Input: part model. Units: mm. Frame: model coordinates. A direction names the side the tool comes from. Coordinates: 2 decimals unless noted, no trailing zeros. Loops run counter-clockwise (first coordinate to the right, second up) from the corner with the lowest first, then second, coordinate; pieces in that order, holes last.
Item 1: Section A-A on x = -2.5. Return loops of the section in (y, z), and give its area (3 significant figures).
Item 2: Contact query for flat-ended pins moving along their axis: P1, Ø0.8, axis at y = 2, z = 1, coming from the +X side; P2, Ø1.5, axis at y = -13.25, z = 2.5, coming from the -X side; P3, Ø1.5, axis at x = -41, z = 0.5, coming from the -Y side. Output: stop coordinate, or through.
Item 3: Reachability of faces 1 (the flat face through (60.5, 12, 1)), 2 (the flat face through (62, -7.5, 4)), 3 (the flat face through (-9.92, -5.79, 2.46)) from +Z, -Z, +X, -X, +Y, -Y: full face, straight path, thin tool, end or side. Return the list, or none.
Item 4: Pull-direction query (Z, two-part tool) for faces 4 (the cylindrical face through (11.1, 15.2, 2.5)), 5 (the flat face through (0, -17, 2.5)), 6 (the cylindrical face through (16.22, -14.98, 2.34)); classes: released by +Z, released by -Z, zero draft, split by the parting line, or undercut.
Item 5: Ray query, line 1 along Y through (x, z) = (58.7, 2.5); line 2 along X through (y, z) = (15, 2.7); line 3 along Z through (x, y) = (-15, 14.75). Return the intervals inside material, ascending.
Item 6: Section B-B on x = 11.05. Return loops of the section in (y, z).
Autodesk Inventor part; units mm, degrees
ref_plane "YZ Plane" through (0, 0, 0) normal (1, 0, 0) x (0, 1, 0)
ref_plane "XZ Plane" through (0, 0, 0) normal (0, 1, 0) x (-1, 0, 0)
ref_plane "XY Plane" through (0, 0, 0) normal (0, 0, 1) x (1, 0, 0)
sketch "スケッチ1" plane through (0, 0, 0) normal (0, 0, 1) x (1, 0, 0)
  line L0 (-60.5, 9.6) -> (-60.5, 16.25)
  line L1 (-60.5, 16.25) -> (-20, 16.25)
  line L2 (20, 16.25) -> (60.5, 16.25)
  line L3 (60.5, 16.25) -> (60.5, 9.6)
  line L4 (0, 0) -> (0, 16.25) construction
  line L5 (0, 0) -> (62.5, 0) construction
  line L6 (60.5, 7.5) -> (62.5, 7.5)
  line L7 (62.5, 7.5) -> (62.5, -7.5)
  line L8 (62.5, -7.5) -> (60.5, -7.5)
  line L9 (-20, -16.25) -> (20, -16.25) construction
  line L10 (20, -16.25) -> (20, 16.25) construction
  line L11 (20, 16.25) -> (-20, 16.25) construction
  line L12 (-20, 16.25) -> (-20, -16.25) construction
  line L13 (-20, -16.25) -> (20, 16.25) construction
  line L14 (20, -16.25) -> (-20, 16.25) construction
  line L15 (-60.5, -16.25) -> (60.5, -16.25) construction
  line L16 (60.5, -16.25) -> (60.5, 16.25) construction
  line L17 (60.5, 16.25) -> (-60.5, 16.25) construction
  line L18 (-60.5, 16.25) -> (-60.5, -16.25) construction
  line L19 (-60.5, -16.25) -> (60.5, 16.25) construction
  line L20 (60.5, -16.25) -> (-60.5, 16.25) construction
  arc A0 (60.5, 9.6) -> (60.5, 7.5) centre (60.5, 8.55) ccw
  arc A1 (60.5, -7.5) -> (60.5, -9.6) centre (60.5, -8.55) ccw
  line L21 (60.5, -9.6) -> (60.5, -16.25)
  line L22 (60.5, -16.25) -> (20, -16.25)
  line L23 (20, -16.25) -> (12.1, -16.25)
  line L24 (-20, 16.25) -> (-12.1, 16.25)
  line L25 (-10, 16.25) -> (-10, 18.25)
  line L26 (-10, 18.25) -> (10, 18.25)
  line L27 (10, 18.25) -> (10, 16.25)
  line L28 (20, 16.25) -> (12.1, 16.25)
  arc A2 (-12.1, 16.25) -> (-10, 16.25) centre (-11.05, 16.25) ccw
  arc A3 (10, 16.25) -> (12.1, 16.25) centre (11.05, 16.25) ccw
  line L29 (-60.5, 7.5) -> (-62.5, 7.5)
  line L30 (-62.5, 7.5) -> (-62.5, -7.5)
  line L31 (-62.5, -7.5) -> (-60.5, -7.5)
  arc A4 (-60.5, 7.5) -> (-60.5, 9.6) centre (-60.5, 8.55) ccw
  arc A5 (-60.5, -9.6) -> (-60.5, -7.5) centre (-60.5, -8.55) ccw
  line L32 (-60.5, -9.6) -> (-60.5, -16.25)
  line L33 (-60.5, -16.25) -> (-20, -16.25)
  line L34 (-20, -16.25) -> (-12.1, -16.25)
  line L35 (-10, -16.25) -> (-10, -18.25)
  line L36 (-10, -18.25) -> (10, -18.25)
  line L37 (10, -18.25) -> (10, -16.25)
  arc A6 (-10, -16.25) -> (-12.1, -16.25) centre (-11.05, -16.25) ccw
  arc A7 (12.1, -16.25) -> (10, -16.25) centre (11.05, -16.25) ccw
  line L38 (-16.55, 19.1799) -> (-13.45, 19.1799) construction
  line L39 (-13.45, 19.1799) -> (-13.45, 12.4242) construction
  line L40 (-13.45, 12.4242) -> (-16.55, 12.4242) construction
  line L41 (-16.55, 12.4242) -> (-16.55, 19.1799) construction
  line L42 (-15, 19.1799) -> (-15, 12.4242) construction
  point P0 (0, 18.25)
  point P1 (0, 0)
  dimension "d0" = 1.05
  dimension "d1" = 32.5
  dimension "d2" = 121
  dimension "d3" = 40
  dimension "d23" = 2
  dimension "d30" = 2
  dimension "d34" = 8.75
  dimension "d53" = 20
  dimension "d54" = 3.1
  dimension "d55" = 5
  dimension "d85" = 32.5
extrude "押し出し1" add sketch "スケッチ1" along normal blind 5
sketch "スケッチ2" plane through (0, 0, 0) normal (0, 0, -1) x (-1, 0, 0)
  line L0 (60.5, 9.6) -> (60.5, 16.25)
  line L1 (-60.5, 16.25) -> (-60.5, 9.6)
  line L2 (-68.6427, 17.3125) -> (-60.5, 17.3125)
  line L3 (-60.5, 17.3125) -> (-60.5, -16.751)
  line L4 (-60.5, -16.751) -> (-68.6427, -16.751)
  line L5 (-68.6427, -16.751) -> (-68.6427, 17.3125)
  line L6 (60.5, 21.1805) -> (66.358, 21.1805)
  line L7 (66.358, 21.1805) -> (66.358, -13.6193)
  line L8 (66.358, -13.6193) -> (60.5, -13.6193)
  line L9 (60.5, -13.6193) -> (60.5, 21.1805)
  line L10 (-20, -16.25) -> (-12.1, -16.25)
  line L11 (-17.1371, 25.1848) -> (11.8342, 25.1848)
  line L12 (11.8342, 25.1848) -> (11.8342, 16.25)
  line L13 (11.8342, 16.25) -> (-17.1371, 16.25)
  line L14 (-17.1371, 16.25) -> (-17.1371, 25.1848)
  line L15 (-13.151, -21.5857) -> (17.7795, -21.5857)
  line L16 (17.7795, -21.5857) -> (17.7795, -16.25)
  line L17 (17.7795, -16.25) -> (-13.151, -16.25)
  line L18 (-13.151, -16.25) -> (-13.151, -21.5857)
  line L19 (-12.1, 16.25) -> (-60.5, 16.25)
  line L20 (-60.5, -16.25) -> (-12.1, -16.25)
  point P0 (0, 0)
extrude "押し出し2" cut sketch "スケッチ2" against normal blind 2.5
sketch "スケッチ3" plane through (12.1, 16.25, 0) normal (0, 1, 0) x (1, 0, 0)
  line L0 (-2.1, 0) -> (-2.1, -5)
  line L1 (-2.1, -5) -> (-22.1, -5) construction
  line L2 (-12.1, -5) -> (-12.1, 7.4607) construction
  line L3 (48.4, 0) -> (48.4, -5)
  point P0 (-12.1, 0)
  point P1 (2.9, -2.5)
  point P2 (-27.1, -2.5)
  point P3 (48.4, -2.5)
  dimension "d60" = 5
hole "穴1" at (15, 16.25, 2.5) at (-15, 16.25, 2.5) direction (0, -1, 0) diameter 2.459 depth 2.5
mirror "ミラー1" about plane through (0, 0, 0) normal (0, 1, 0) of "穴1"
sketch "スケッチ4" plane through (60.5, -16.25, 5) normal (1, 0, 0) x (0, 0, -1)
  line L0 (5, 16.25) -> (0, 16.25) construction
  line L1 (0, 23.75) -> (0, 8.75) construction
  line L2 (5, 6.65) -> (0, 6.65)
  line L3 (5, 0) -> (0, 0)
  point P0 (2.5, 3)
  point P1 (2.5, 29.5)
  point P2 (2.5, 6.65)
  dimension "d86" = 3
  dimension "d87" = 26.5
hole "穴2" at (60.5, -13.25, 2.5) at (60.5, 13.25, 2.5) direction (-1, 0, 0) diameter 2.459 depth 2.5
mirror "ミラー2" about plane through (0, 0, 0) normal (1, 0, 0) of "穴2"
sketch "スケッチ5" plane through (0, 0, 0) normal (0, 0, -1) x (-1, 0, 0)
  line L0 (10, 16.25) -> (-10, 16.25)
  line L1 (-60.5, 7.5) -> (-60.5, 9.6)
  line L2 (-30.5, -11.25) -> (30.5, -11.25) construction
  line L3 (30.5, -11.25) -> (30.5, 11.25) construction
  line L4 (30.5, 11.25) -> (-30.5, 11.25) construction
  line L5 (-30.5, 11.25) -> (-30.5, -11.25) construction
  line L6 (-30.5, -11.25) -> (30.5, 11.25) construction
  line L7 (30.5, -11.25) -> (-30.5, 11.25) construction
  line L8 (-30.5, 9.1183) -> (-30.5, -9.1183)
  line L9 (-30.5, -9.1183) -> (-5.7793, 0)
  line L10 (-5.7793, 0) -> (-30.5, 9.1183)
  line L11 (-24.7207, 11.25) -> (24.7207, 11.25)
  line L12 (24.7207, 11.25) -> (0, 2.1317)
  line L13 (0, 2.1317) -> (-24.7207, 11.25)
  line L14 (-24.7207, -11.25) -> (24.7207, -11.25)
  line L15 (24.7207, -11.25) -> (0, -2.1317)
  line L16 (0, -2.1317) -> (-24.7207, -11.25)
  line L17 (30.5, 9.1183) -> (30.5, -9.1183)
  line L18 (30.5, -9.1183) -> (5.7793, 0)
  line L19 (5.7793, 0) -> (30.5, 9.1183)
  point P0 (-12.1, 16.25)
  point P1 (-20, 16.25)
  point P2 (-60.5, 16.25)
  point P3 (0, 0)
  dimension "d76" = 5
  dimension "d77" = 30
  dimension "d78" = 4
  dimension "d79" = 4
  dimension "d80" = 4
  dimension "d81" = 4
extrude "押し出し3" cut sketch "スケッチ5" against normal blind 10
fillet "フィレット1" radius 1.05 12 edges at (30.5, 9.1183, 2.5) (30.5, -9.1183, 2.5) (24.7207, 11.25, 2.5) (5.7793, 0, 2.5) (0, -2.1317, 2.5) (0, 2.1317, 2.5) (-30.5, -9.1183, 2.5) (24.7207, -11.25, 2.5) (-30.5, 9.1183, 2.5) (-24.7207, 11.25, 2.5) (-24.7207, -11.25, 2.5) (-5.7793, 0, 2.5)
equation "\"d85\" = d1"
equation "\"d79\" = d78"
equation "\"d80\" = d79"
equation "\"d81\" = d78"
equation "\"d48\" = 26.5"
equation "\"d52\" = 5"
properties part number "Trunk_chest_back_forth_frame" material "アセタール樹脂、黒"
Results found:
1. outline: (-18.25, 2.5) - (-16.25, 2.5) - (-16.25, 0) - (-11.25, 0) - (-11.25, 5) - (-18.25, 5) - close; (-3.05, 0) - (3.05, 0) - (3.05, 5) - (-3.05, 5) - close; (11.25, 0) - (16.25, 0) - (16.25, 2.5) - (18.25, 2.5) - (18.25, 5) - (11.25, 5) - close
1. area: 90.5 mm2
2. P1: stops at x = 60.5
2. P2: stops at x = -58
2. P3: stops at y = -16.25
3. face 1: +Z, -Z, +X, +Y
3. face 2: +Z, -Z, +X, -Y
3. face 3: +Z, -Z
4. face 4: zero draft
4. face 5: released by -Z
4. face 6: undercut
5. line 1: y = -16.25 to -14.48, -12.02 to 12.02, 14.48 to 16.25
5. line 2: x = -60.5 to -16.21, -13.79 to 13.79, 16.21 to 60.5
5. line 3: z = 0 to 1.27, 3.73 to 5
6. outline: (-15.2, 0) - (-11.25, 0) - (-11.25, 5) - (-15.2, 5) - close; (-6.21, 0) - (-1.94, 0) - (-1.94, 5) - (-6.21, 5) - close; (1.94, 0) - (6.21, 0) - (6.21, 5) - (1.94, 5) - close; (11.25, 0) - (15.2, 0) - (15.2, 5) - (11.25, 5) - close
